```python
from build123d import *

# Parameters (mm, degrees)
F0_R     = 12.65
F1_DEPTH = 15
F2_T     = -2
F3_SIZE  = 1.5


with BuildPart() as f1:
    # F0 (on Top) → F1 (new body)
    with BuildSketch(Plane.XY):
        Circle(F0_R)
    extrude(amount=F1_DEPTH)

    # F2
    f2_openings = [f1.faces().sort_by_distance(p)[0] for p in [
        (0, 0, 15),
    ]]
    offset(amount=F2_T, openings=f2_openings)

    # F3
    f3_edges = [f1.edges().sort_by_distance(p)[0] for p in [
        (-10.65, 0, 15),
    ]]
    chamfer(f3_edges, length=F3_SIZE)


solid = f1.part
```
Geometry: final body of the model. Coordinates: model frame, mm. A direction names the side the tool comes from. Round coordinates to 2 decimals unless told otherwise and drop trailing zeros. Loops run counter-clockwise (first coordinate to the right, second up) from the corner with the lowest first, then second, coordinate; pieces in that order, holes last. Notation, with made-up numbers: (29.25, -36.75) -> (49.25, -36.75) arc R11 ccw to (49.25, -19.75) -> close; hole circle Ø11 at (-23.75, 52.5). An arc over 180 degrees is marked (long way). Use one line per item in the form item = value. Start each with the question number.
1) Access query for faces 1 (the flat face through (0, 0, 0)), 2 (the cylindrical face through (10.158, 3.199, 7.67)). Directions: +Z, -Z, +X, -X, +Y, -Y. A direction counts if a zero-diameter tool reaches every point of the face in a straight line with its end or side. Return the directions, or none.
2) Draft query along X for faces 3 (the cylindrical face through (-2.74, -12.35, 7.4)), 4 (the flat face through (-6.6, 10.4, 15)), 5 (the flat face through (0, 0, 2)). Return one class per face: released by +X, released by -X, zero draft, split by the parting line, or undercut.
3) Line query: L1, parallel to Y at x = 0, z = 6.75; L2, parallel to Z at x = -3, y = 4; L3, parallel to Y at x = 8.5, z = 4.75. Output: solid intervals per line, ascending.
4) Section B-B on z = 6.25. Output: boundary loops of the cut face in (x, y), then the cut area to 3 significant figures.
5) First-contact query: P1, Ø5, axis at y = -6.5, z = 7.5, coming from the -X side; P2, Ø3, axis at x = 4, z = 4, coming from the +Y side; P3, Ø1, axis at x = 9, z = 9.5, coming from the -Y side. Flat tips, straight axial feed; report the tip coordinate or a pass-through.
6) Section A-A on x = 0. Output: boundary loops of the cut face in (y, z).
Response:
q1.face_1 = -Z, +X, -X, +Y, -Y
q1.face_2 = +Z
q2.face_3 = split by the parting line
q2.face_4 = zero draft
q2.face_5 = undercut
q3.L1 = -12.65 to -10.65, 10.65 to 12.65
q3.L2 = 0 to 2
q3.L3 = -9.37 to -6.42, 6.42 to 9.37
q4.outline = circle Ø25.3 at (0, 0); hole circle Ø21.3 at (0, 0)
q4.area = 146 mm^2
q5.P1 = -12
q5.P2 = 12.4
q5.P3 = -9.37
q6.outline = (-12.65, 0) -> (12.65, 0) -> (12.65, 15) -> (12.15, 15) -> (10.65, 13.5) -> (10.65, 2) -> (-10.65, 2) -> (-10.65, 13.5) -> (-12.15, 15) -> (-12.65, 15) -> close
